from build123d import *

# Parameters (mm, degrees)
SKETCH1_R           = 12.5
BOSS_EXTRUDE1_DEPTH = 7.5
SKETCH2_W           = 35
SKETCH2_H           = 8.580767914
BOSS_EXTRUDE2_DEPTH = 25
SKETCH3_W           = 25
SKETCH3_H           = 8.580767914
CUT_EXTRUDE1_DEPTH  = 20
SKETCH4_R           = 2.5
BOSS_EXTRUDE3_DEPTH = 5
SKETCH5_R           = 2.5
BOSS_EXTRUDE4_DEPTH = 5
CHAMFER1_SIZE       = 5
CHAMFER2_SIZE       = 5


with BuildPart() as part:
    # Sketch1 → Boss-Extrude1 (new body)
    with BuildSketch(Plane(origin=(0, 0, 0), x_dir=(1, 0, 0), z_dir=(0, 1, 0))):
        Circle(SKETCH1_R)
    extrude(amount=BOSS_EXTRUDE1_DEPTH)

    # Sketch2 → Boss-Extrude2 (add)
    with BuildSketch(Plane(origin=(0, 7.5, 0), x_dir=(1, 0, 0), z_dir=(0, 1, 0))):
        Rectangle(SKETCH2_W, SKETCH2_H)
    extrude(amount=BOSS_EXTRUDE2_DEPTH)

    # Sketch3 → Cut-Extrude1 (cut)
    with BuildSketch(Plane(origin=(0, 32.5, 0), x_dir=(1, 0, 0), z_dir=(0, 1, 0))):
        Rectangle(SKETCH3_W, SKETCH3_H)
    extrude(amount=-CUT_EXTRUDE1_DEPTH, mode=Mode.SUBTRACT)

    # Sketch4 → Boss-Extrude3 (add)
    with BuildSketch(Plane(origin=(-12.5, 0, 0), x_dir=(0, 0, -1), z_dir=(1, 0, 0))):
        with Locations((0, 27.5)):
            Circle(SKETCH4_R)
    extrude(amount=BOSS_EXTRUDE3_DEPTH)

    # Sketch5 → Boss-Extrude4 (add)
    with BuildSketch(Plane.ZY.offset(-12.5)):
        with Locations((0, 27.5)):
            Circle(SKETCH5_R)
    extrude(amount=BOSS_EXTRUDE4_DEPTH)

    # Chamfer1
    chamfer1_edges = [part.edges().sort_by_distance(p)[0] for p in [
        (-12.5, 12.5, 0),
    ]]
    chamfer(chamfer1_edges, length=CHAMFER1_SIZE)

    # Chamfer2
    chamfer2_edges = [part.edges().sort_by_distance(p)[0] for p in [
        (12.5, 12.5, 0),
    ]]
    chamfer(chamfer2_edges, length=CHAMFER2_SIZE)


solid = part.part
The listing builds one solid part. Answer for the finished solid, in the listing's coordinates (mm). A direction names the side the tool comes from. Coordinates: 2 decimals unless noted, no trailing zeros. Write each loop counter-clockwise with the first axis right and the second up, starting at its lowest first coordinate (ties: lowest second). Pieces come first, ordered by that corner, then holes. Notation, with made-up numbers: (80, 62.5) - (118, 62.5) arc R23 ccw to (118, 99.5) - close; hole circle Ø9 at (51, 74). An arc over 180 degrees is marked (long way). Return JSON: item names as keys, results as strings.
1. Each of these flat-tipped pins is pushed along its axis until it touches: pin 1 Ø1.5 at (y, z) = (20, -6) entering from -X; pin 2 Ø10 at (x, z) = (-14, -5.5) entering from +Y; pin 3 Ø9 at (x, z) = (0.5, 9) entering from +Y; pin 4 Ø4.5 at (x, z) = (-15.5, -2) entering from -Y. Where does it stop, or does it pass through?
Final values:
{"pin 1": "through", "pin 2": "y = 32.5", "pin 3": "y = 7.5", "pin 4": "y = 7.5"}
2. Consider line 1 along X through (y, z) = (31, 2); line 2 along Y through (x, z) = (-7, -2.75); line 3 along Y through (x, z) = (-3, -5.25). Determine where each line is inside the solid, lowest interval first.
Final values:
{"line 1": "-17.5 to -12.5, 12.5 to 17.5", "line 2": "0 to 12.5", "line 3": "0 to 7.5"}
3. Which of the six approach directions +Z, -Z, +X, -X, +Y, -Y give full straight-line access (tool end or side, diameter ignored) to faces 1 (the face through (0, 7.5, 7)), 2 (the face through (11.923, 3.698, -3.755)), 3 (the face through (-7.5, 28, 0))?
Final values:
{"face 1": "+Z, +X, -X, +Y", "face 2": "-Y", "face 3": "+Z, -Z, +Y"}
4. The part is cut by section B-B on z = 0. Determine the outline of the cut face in (x, y), then the cut area to 4 significant figures.
Final values:
{"outline": "(-17.5, 7.5) - (-12.5, 7.5) - (-12.5, 0) - (12.5, 0) - (12.5, 7.5) - (17.5, 7.5) - (17.5, 32.5) - (12.5, 32.5) - (12.5, 30) - (7.5, 30) - (7.5, 25) - (12.5, 25) - (12.5, 17.5) - (7.5, 12.5) - (-7.5, 12.5) - (-12.5, 17.5) - (-12.5, 25) - (-7.5, 25) - (-7.5, 30) - (-12.5, 30) - (-12.5, 32.5) - (-17.5, 32.5) - close", "area": "637.5 mm^2"}
5. The part is cut by section C-C on x = -9. Determine the outline of the cut face in (y, z), then the cut area to 3 significant figures.
Final values:
{"outline": "(0, -8.67) - (7.5, -8.67) - (7.5, -4.29) - (14, -4.29) - (14, 4.29) - (7.5, 4.29) - (7.5, 8.67) - (0, 8.67) - close; circle Ø5 at (27.5, 0)", "area": "206 mm^2"}
6. The part is cut by section D-D on x = 0. Determine the outline of the cut face in (y, z).
Final values:
{"outline": "(0, -12.5) - (7.5, -12.5) - (7.5, -4.29) - (12.5, -4.29) - (12.5, 4.29) - (7.5, 4.29) - (7.5, 12.5) - (0, 12.5) - close"}
7. For a pull along Y with two mould halves and no side action, classify faces 4 (the face through (-10, 15, 0)), 5 (the face through (-15, 7.5, 0)), 6 (the face through (17.5, 20, 0)) as +Y half, -Y half, draft (parallel to the pull), parting line (faces both ways), or undercut.
Final values:
{"face 4": "undercut", "face 5": "-Y half", "face 6": "draft"}
8. The part is cut by section A-A on y = 21. Determine the outline of the cut face in (x, z), then the cut area to 3 significant figures.
Final values:
{"outline": "(-17.5, -4.29) - (-12.5, -4.29) - (-12.5, 4.29) - (-17.5, 4.29) - close; (12.5, -4.29) - (17.5, -4.29) - (17.5, 4.29) - (12.5, 4.29) - close", "area": "85.8 mm^2"}
